Could you check a few things on this model? Use its own coordinates, in mm. Face numbers are marked on the shaded views. Give positions to 0.01 mm unless a question says otherwise; leave off trailing zeros. Order: outer loops, then holes, each group sorted by start corner. A loop starts at its lowest first (then second) coordinate and runs counter-clockwise, first axis right, second up. Notation, with made-up numbers: (73.5, -13) - (92.5, -13) arc R15 ccw to (92.5, 11) - close; hole circle Ø7 at (63, -5.75). An arc over 180 degrees is marked (long way). One line per question, with ' | ' between items. Start each with the question number.
1. I need wall thicknesses on probe 1 along Y at (x, z) = (10, -0.25); probe 2 along X at (y, z) = (-0.35, -0.6); probe 3 along X at (y, z) = (0.1, -0.45). Which ranges of each line are inside material? Lowest first, please. Write a range as from..to.
2. Imagine slicing it at A-A (x = 10). Please give me the cut outline in (y, z).
3. If we mould it in two halves opening along Y, with no side actions, what happens to the marked faces 1, 2 and 3? For each: released by +Y, released by -Y, zero draft, split by the parting line, or undercut.
4. Imagine slicing it at C-C (z = 0.25). Please give me the cut outline in (x, y), and give its area (3 significant figures).
5. Imagine slicing it at D-D (x = 6). Please give me the cut outline in (y, z).
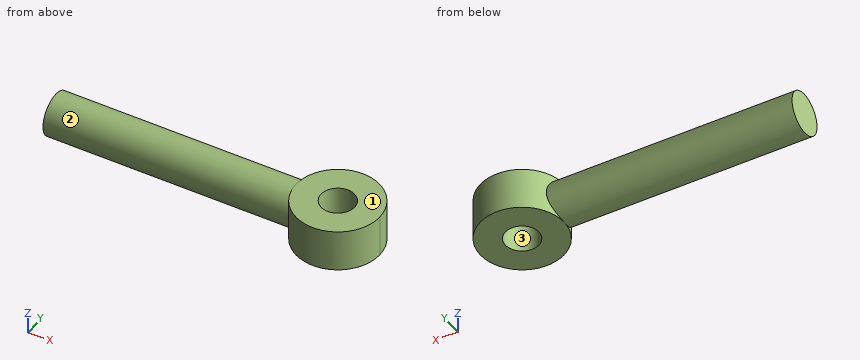
```python
from build123d import *
from build123d.topology import SkipClean

# Parameters (mm, degrees)
SKETCH1_R                = 0.75
BOSS_EXTRUDE1_DEPTH      = 10
BOSS_EXTRUDE2_DEPTH      = 0.75
BOSS_EXTRUDE2_DEPTH_BACK = 0.75
SKETCH2_R                = 1.5
SKETCH3_R                = 0.6
CUT_EXTRUDE1_DEPTH       = 1.5


with BuildPart() as part:
    # Sketch1 → Boss-Extrude1 (new body)
    with BuildSketch(Plane(origin=(0, 0, 0), x_dir=(0, 0, -1), z_dir=(1, 0, 0))):
        Circle(SKETCH1_R)
    extrude(amount=BOSS_EXTRUDE1_DEPTH)

    # Sketch2 → Boss-Extrude2 (add, two sides: drawn at the far end of the back side and taken through both)
    with SkipClean():  # the faces are left unmerged after this step: merging them gives an invalid solid
        with BuildSketch(Plane.XY.offset(-BOSS_EXTRUDE2_DEPTH_BACK)):
            with Locations((10, 0)):
                Circle(SKETCH2_R)
        extrude(amount=BOSS_EXTRUDE2_DEPTH + BOSS_EXTRUDE2_DEPTH_BACK)

    # Sketch3 → Cut-Extrude1 (cut)
    with SkipClean():  # the faces are left unmerged after this step: merging them gives an invalid solid
        with BuildSketch(Plane.XY.offset(0.75)):
            with Locations((10, 0)):
                Circle(SKETCH3_R)
        extrude(amount=-CUT_EXTRUDE1_DEPTH, mode=Mode.SUBTRACT)


solid = part.part
```
Results found:
1) probe 1: y = -1.5..-0.6, 0.6..1.5 | probe 2: x = 0..9.51, 10.49..11.46 | probe 3: x = 0..9.41, 10.59..11.5
2) outline: (-1.5, -0.75) - (-0.6, -0.75) - (-0.6, 0.75) - (-1.5, 0.75) - close; (0.6, -0.75) - (1.5, -0.75) - (1.5, 0.75) - (0.6, 0.75) - close
3) face 1: zero draft | face 2: split by the parting line | face 3: undercut
4) outline: (0, -0.71) - (8.68, -0.71) arc R1.5 ccw (long way) to (8.68, 0.71) - (0, 0.71) - close; hole circle Ø1.2 at (10, 0) | area: 18.0 mm2
5) outline: circle Ø1.5 at (0, 0)
